For this review, take the finished solid that the model builds, in its own axes (mm). Coordinates: 2 decimals unless noted, no trailing zeros. Loops run counter-clockwise (first coordinate to the right, second up) from the corner with the lowest first, then second, coordinate; pieces in that order, holes last.
```python
from build123d import *

# Parameters (mm, degrees)
SKETCH1_W           = 120
SKETCH1_H           = 67.6
SKETCH1_W_2         = 200
SKETCH1_H_2         = 300
BOSS_EXTRUDE1_DEPTH = 5
CHAMFER1_SIZE       = 40


with BuildPart() as part:
    # Sketch1 → Boss-Extrude1 (new body)
    with BuildSketch(Plane.XY):
        with Locations((0, 358.8)):
            Rectangle(SKETCH1_W, SKETCH1_H)
        with Locations((-160, 175)):
            Rectangle(SKETCH1_W_2, SKETCH1_H_2)
        with Locations((0, 175)):
            Rectangle(SKETCH1_W, SKETCH1_H_2)
        with Locations((160, 175)):
            Rectangle(SKETCH1_W_2, SKETCH1_H_2)
        with Locations((0, -8.8)):
            Rectangle(SKETCH1_W, SKETCH1_H)
    extrude(amount=BOSS_EXTRUDE1_DEPTH)

    # Chamfer1
    chamfer1_edges = [part.edges().sort_by_distance(p)[0] for p in [
        (260, 325, 2.5),
        (260, 25, 2.5),
        (-260, 25, 2.5),
        (-260, 325, 2.5),
    ]]
    chamfer(chamfer1_edges, length=CHAMFER1_SIZE)


solid = part.part
```
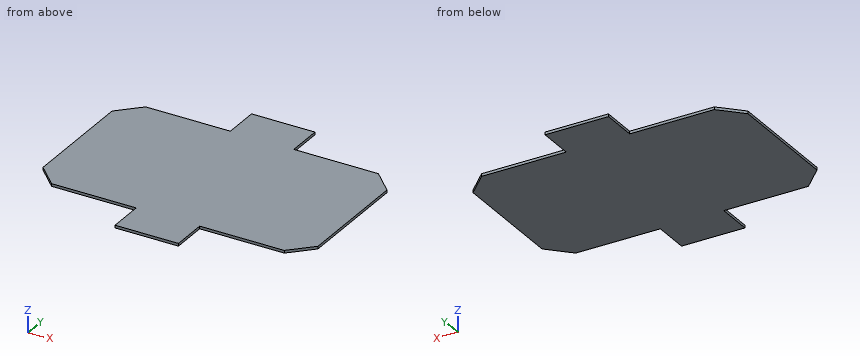
Q1. Wall thickness on probe 1 along Y at (x, z) = (-143.5, 4.65); probe 2 along X at (y, z) = (16.5, 2); probe 3 along X at (y, z) = (43.5, 2.25): over which ranges is each line inside the solid? List them lowest first.
Q2. Consider section C-C (x = -69). State the section outline as (y, z) points.
Q3. For pin 1 Ø6 at (x, y) = (188.5, 320.5) entering from -Z; pin 2 Ø3 at (x, z) = (185, 2) entering from -Y; pin 3 Ø1.5 at (x, z) = (-166.5, 2.5) entering from +Y; pin 4 Ø2.5 at (y, z) = (374, 3) entering from +X, all flat-tipped, find the tip position at first contact; note any pin that passes through.
Q4. Consider section B-B (y = 44). State the section outline as (x, z) points.
Q5. Consider section A-A (z = 1.55). State the section outline as (x, y) points.
Model answer:
1. probe 1: y = 25 to 325
1. probe 2: x = -60 to 60
1. probe 3: x = -238.5 to 238.5
2. outline: (25, 0) - (325, 0) - (325, 5) - (25, 5) - close
3. pin 1: stops at z = 0
3. pin 2: stops at y = 25
3. pin 3: stops at y = 325
3. pin 4: stops at x = 60
4. outline: (-239, 0) - (239, 0) - (239, 5) - (-239, 5) - close
5. outline: (-260, 65) - (-220, 25) - (-60, 25) - (-60, -42.6) - (60, -42.6) - (60, 25) - (220, 25) - (260, 65) - (260, 285) - (220, 325) - (60, 325) - (60, 392.6) - (-60, 392.6) - (-60, 325) - (-220, 325) - (-260, 285) - close
